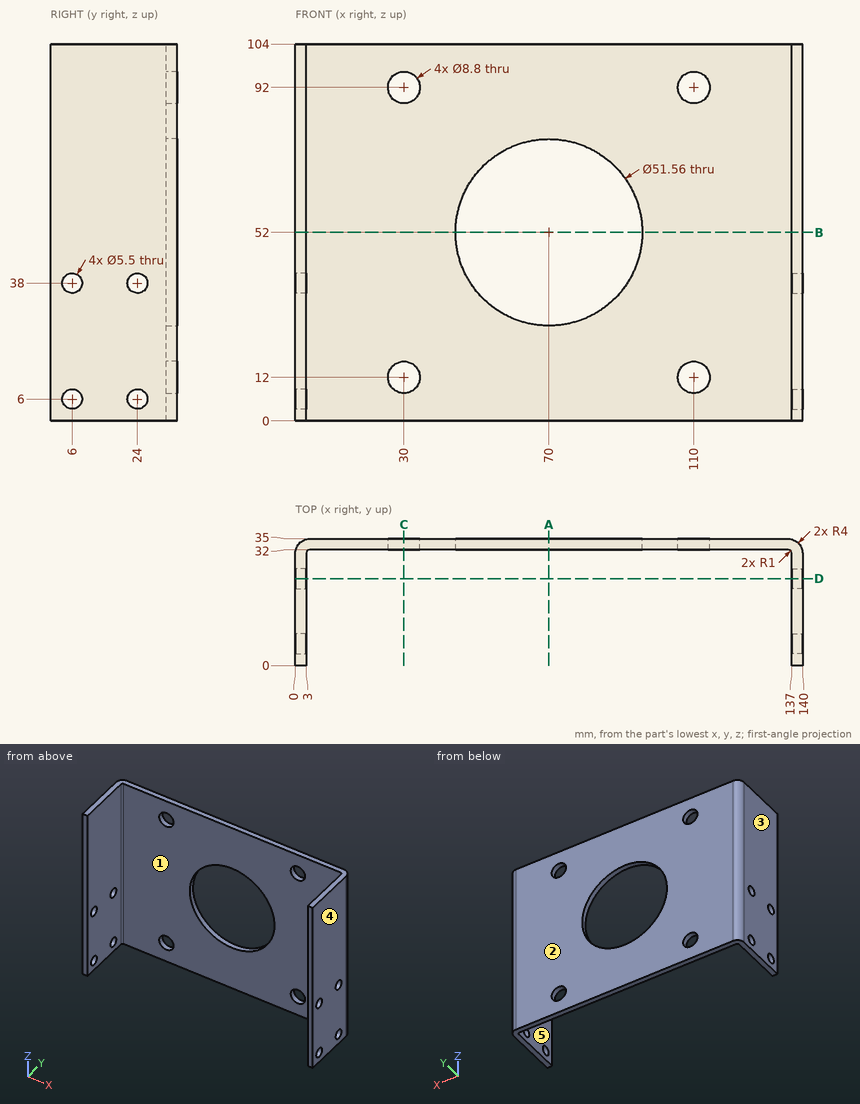
Job drawing, mm, ordinate dimensions from the low corner. One solid piece. A direction names the side the tool comes from. Round coordinates to 2 decimals unless told otherwise and drop trailing zeros. Loops run counter-clockwise (first coordinate to the right, second up) from the corner with the lowest first, then second, coordinate; pieces in that order, holes last. Notation, with made-up numbers: (3.5, 66.25) -> (53.5, 66.25) arc R18 cw to (53.5, 100.25) -> close; hole circle Ø9 at (-31, 45.5). An arc over 180 degrees is marked (long way). One line per item, written item: value. Start each with the question number.
Q1. Drop flat-ended pins along their axis: pin 1 Ø8 at (x, z) = (110, 92) entering from -Y; pin 2 Ø7 at (y, z) = (6, 6) entering from -X; pin 3 Ø4 at (x, z) = (121.5, 44.5) entering from -Y. Give the stop position or say it passes through.
Q2. Cut at A-A on x = 70. List the corners of the cut face in (y, z), plus the area to 3 significant figures.
Q3. 3-axis set-ups, long thin cutter, end or side, ignore diameter. For the marked faces 1 and 2: which of +Z, -Z, +X, -X, +Y, -Y reach the whole face in a straight line?
Q4. Two-plate mould, pull along X, no slides. Class the marked faces 3, 4 and 5: released by +X, released by -X, zero draft, split by the parting line, or undercut.
Q5. Cut at D-D on y = 24. List the corners of the cut face in (x, z), plus the area to 3 significant figures.
Q6. Cut at C-C on x = 30. List the corners of the cut face in (y, z), plus the area to 3 significant figures.
Q7. Probe line 1 along Z through (x, y) = (2.35, 24); line 2 along X through (y, z) = (8.5, 89); line 3 along X through (y, z) = (32.5, 35.5). List the from-to ranges inside material, lowest first.
Q8. Cut at B-B on z = 52. List the corners of the cut face in (x, y).
Computed:
1. pin 1: through
1. pin 2: x = 0
1. pin 3: y = 32
2. outline: (32, 0) -> (35, 0) -> (35, 26.22) -> (32, 26.22) -> close; (32, 77.78) -> (35, 77.78) -> (35, 104) -> (32, 104) -> close
2. area: 157 mm²
3. face 1: +Z, -Z, -Y
3. face 2: +Z, -Z, +X, -X, +Y
4. face 3: released by -X
4. face 4: released by +X
4. face 5: undercut
5. outline: (0, 0) -> (3, 0) -> (3, 3.25) -> (0, 3.25) -> close; (0, 8.75) -> (3, 8.75) -> (3, 35.25) -> (0, 35.25) -> close; (0, 40.75) -> (3, 40.75) -> (3, 104) -> (0, 104) -> close; (137, 0) -> (140, 0) -> (140, 3.25) -> (137, 3.25) -> close; (137, 8.75) -> (140, 8.75) -> (140, 35.25) -> (137, 35.25) -> close; (137, 40.75) -> (140, 40.75) -> (140, 104) -> (137, 104) -> close
5. area: 558 mm²
6. outline: (32, 0) -> (35, 0) -> (35, 7.6) -> (32, 7.6) -> close; (32, 16.4) -> (35, 16.4) -> (35, 87.6) -> (32, 87.6) -> close; (32, 96.4) -> (35, 96.4) -> (35, 104) -> (32, 104) -> close
6. area: 259 mm²
7. line 1: 0 to 3.25, 8.75 to 35.25, 40.75 to 104
7. line 2: 0 to 3, 137 to 140
7. line 3: 0.29 to 50.19, 89.81 to 139.71
8. outline: (0, 0) -> (3, 0) -> (3, 31) arc R1 cw to (4, 32) -> (44.22, 32) -> (44.22, 35) -> (4, 35) arc R4 ccw to (0, 31) -> close; (95.78, 32) -> (136, 32) arc R1 cw to (137, 31) -> (137, 0) -> (140, 0) -> (140, 31) arc R4 ccw to (136, 35) -> (95.78, 35) -> close
